from build123d import *

# Parameters (mm, degrees)
SKETCH1_R           = 1.5875
BOSS_EXTRUDE1_DEPTH = 31.75
SKETCH2_W           = 6.35
SKETCH2_H           = 12.7
CUT_EXTRUDE1_DEPTH  = 12.863329641


with BuildPart() as part:
    # Sketch1 → Boss-Extrude1 (new body)
    with BuildSketch(Plane(origin=(0, 0, 0), x_dir=(1, 0, 0), z_dir=(0, 1, 0))):
        Polygon((12.7, -6.35), (31.75, -6.35), (64.103560113, -0.64519443), (63.017646158, 5.513329641), (31.75, 0), (0, 0), (0, -3.175), (12.7, -3.175), align=None)
        with Locations((25.4, -3.175)):
            Circle(SKETCH1_R, mode=Mode.SUBTRACT)
    extrude(amount=BOSS_EXTRUDE1_DEPTH)

    # Sketch2 → Cut-Extrude1 (cut, through all)
    with BuildSketch(Plane.XY.offset(6.35)):
        with Locations((18.25625, 15.875)):
            Rectangle(SKETCH2_W, SKETCH2_H)
    extrude(amount=-CUT_EXTRUDE1_DEPTH, mode=Mode.SUBTRACT)


solid = part.part
The model under review builds one solid part; all positions refer to its coordinate system, in mm. A direction names the side the tool comes from. Coordinates: 2 decimals unless noted, no trailing zeros. Write each loop counter-clockwise with the first axis right and the second up, starting at its lowest first coordinate (ties: lowest second). Pieces come first, ordered by that corner, then holes. Notation, with made-up numbers: (88, 25) -> (136, 25) arc R7 cw to (136, 37) -> close; hole circle Ø2 at (-35, 78). An arc over 180 degrees is marked (long way). Answer in a Markdown table with one row per item.
1. We need section B-B, the plane x = 25.4. State the section outline as (y, z) points.
Answers below:
| item | result |
|---|---|
| outline | (0, 0) -> (31.75, 0) -> (31.75, 1.59) -> (0, 1.59) -> close; (0, 4.76) -> (31.75, 4.76) -> (31.75, 6.35) -> (0, 6.35) -> close |
2. Wall thickness on probe 1 along Z at (x, y) = (4, 8.5) (3 decimals); probe 2 along Z at (x, y) = (20.5, 3); probe 3 along Z at (x, y) = (25, 15): over which ranges is each line inside the solid? List them lowest first. Write a range as [from, to].
Answers below:
| item | result |
|---|---|
| probe 1 | z = [0, 3.175] |
| probe 2 | z = [0, 6.35] |
| probe 3 | z = [0, 1.64], [4.71, 6.35] |
3. Clearance check with flat-ended pins moving along their axes: pin 1 Ø7 at (x, z) = (20, 2) entering from -Y; pin 2 Ø14 at (x, y) = (5.5, 15.5) entering from +Z (3 decimals); pin 3 Ø2 at (x, y) = (39.5, 11) entering from +Z; pin 4 Ø12 at (x, y) = (39, 6) entering from -Z. State where each tip first meets the part, or that it passes through.
Answers below:
| item | result |
|---|---|
| pin 1 | stops at y = 0 |
| pin 2 | stops at z = 3.175 |
| pin 3 | stops at z = 5.16 |
| pin 4 | stops at z = -2.34 |
4. For faces 1 (the flat face through (21.431, 16, 3)), 2 (the flat face through (13, 16, 0)), 3 (the flat face through (6, 16, 3.175)), list the 3-axis set-ups (+Z, -Z, +X, -X, +Y, -Y) from which the entire face can be reached by the end or side of a thin tool; tool diameter is ignored.
Answers below:
| item | result |
|---|---|
| face 1 | +Z, -Z |
| face 2 | -Z, -X, +Y, -Y |
| face 3 | +Z, -X, +Y, -Y |
5. We need section D-D, the plane z = -1.5. State the section outline as (x, y) points.
Answers below:
| item | result |
|---|---|
| outline | (40.26, 0) -> (63.73, 0) -> (63.73, 31.75) -> (40.26, 31.75) -> close |
6. We need section A-A, the plane y = 10.5. Give the number of separate pieces and of enclosed holes in the cut face, and give its area (3 significant figures).
Answers below:
| item | result |
|---|---|
| separate pieces | 2 |
| enclosed holes | 1 |
| area | 315 mm^2 |
7. Draft analysis for pull direction Y (two halves, no side actions). For faces 4 (the flat face through (32, 0, 2)), 5 (the flat face through (18, 9.525, 3)), 6 (the cylindrical face through (26.866, 15.653, 3.783)), state which applies: +Y half, -Y half, draft (parallel to the pull), parting line (faces both ways), or undercut.
Answers below:
| item | result |
|---|---|
| face 4 | -Y half |
| face 5 | undercut |
| face 6 | draft |
